The model under review builds one solid part; all positions refer to its coordinate system, in mm. Face numbers are marked on the shaded views. A direction names the side the tool comes from. Coordinates: 2 decimals unless noted, no trailing zeros. Order: outer loops, then holes, each group sorted by start corner. A loop starts at its lowest first (then second) coordinate and runs counter-clockwise, first axis right, second up. Notation, with made-up numbers: M 0,9 L 31,9 A31 ccw 31,35 Z; hole C 8,24.5 d1. An arc over 180 degrees is marked long. Answer as CSV lines item,"result". Start each with the question number.
Q1. Wall thickness on L1, parallel to Z at x = 194, y = 0; L2, parallel to Y at x = 96.5, z = 0; L3, parallel to Y at x = 192, z = -89.5: over which ranges is each line inside the solid? List them lowest first. Write a range as [from, to].
Q2. Consider section A-A on x = 111. Write out the cut boundary in (y, z).
Q3. Consider section B-B on z = -43. Write out the cut boundary in (x, y).
Q4. Machinability: for the marked faces 1 and 2, which of the approach directions +Z, -Z, +X, -X, +Y, -Y give a long, thin tool a straight path to every point of the face, cutting with its end or side? Answer none if there is none.
Q5. For P1, Ø1.5, axis at x = 252, z = -20, coming from the -Y side; P2, Ø2, axis at x = 225, y = -4.5, coming from the +Z side; P3, Ø1.5, axis at x = 195.5, y = -5, coming from the +Z side, all flat-tipped, find the tip position at first contact; note any pin that passes through.
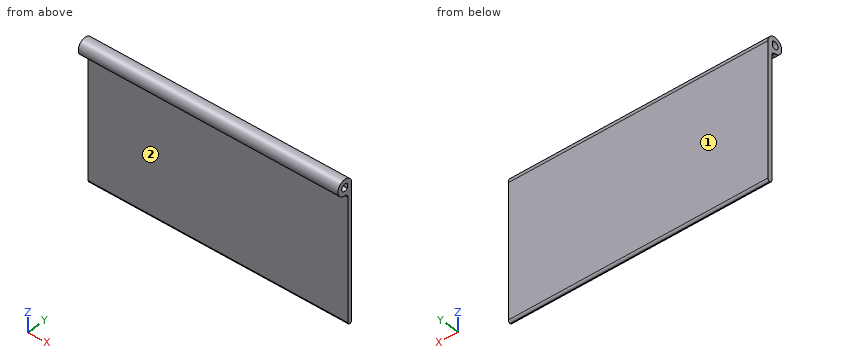
from build123d import *

# Parameters (mm, degrees)
SKETCH1_R               = 9
BOSS_EXTRUDE1_DEPTH     = 300
CUT_EXTRUDE1_DEPTH      = 301.269878609
CUT_EXTRUDE1_DEPTH_BACK = 301.269878609
BOSS_EXTRUDE2_START     = -300
BOSS_EXTRUDE2_DEPTH     = 300
CUT_EXTRUDE2_START      = -300
CUT_EXTRUDE2_DEPTH      = 300


# Read off the part's stored shape, not the designer's step: Cut-Extrude2
with BuildPart() as part:
    # Sketch1 → Boss-Extrude1 (new body)
    with BuildSketch(Plane(origin=(0, 0, 0), x_dir=(0, 0, -1), z_dir=(1, 0, 0))):
        Circle(SKETCH1_R)
    extrude(amount=BOSS_EXTRUDE1_DEPTH)

    # Sketch2 → Cut-Extrude1 (cut, two sides: drawn at the far end of the back side and taken through both)
    with BuildSketch(Plane(origin=(300, 0, 0), x_dir=(0, 0, -1), z_dir=(1, 0, 0)).offset(-CUT_EXTRUDE1_DEPTH_BACK)):
        with BuildLine():
            Line((-2.563201124, 3.2), (2.563201124, 3.2))
            ThreePointArc((2.563201124, 3.2), (0, -4.1), (-2.563201124, 3.2))
        make_face()
    extrude(amount=CUT_EXTRUDE1_DEPTH + CUT_EXTRUDE1_DEPTH_BACK, mode=Mode.SUBTRACT)

    # Sketch3 → Boss-Extrude2 (add)
    with BuildSketch(Plane(origin=(300, 0, 0), x_dir=(0, 0, -1), z_dir=(1, 0, 0)).offset(BOSS_EXTRUDE2_START)):
        with BuildLine():
            ThreePointArc((8.062257748, 4), (8.762428879, 2.054224947), (9, 0))
            ThreePointArc((9, 0), (10.171572875, 2.828427125), (13, 4))
            Line((13, 4), (8.062257748, 4))
        make_face()
        with BuildLine():
            ThreePointArc((5, 4), (7.828427125, 2.828427125), (9, 0))
            ThreePointArc((9, 0), (8.762428879, 2.054224947), (8.062257748, 4))
            Line((8.062257748, 4), (5, 4))
        make_face()
        with BuildLine():
            Line((154, 9), (0, 9))
            ThreePointArc((0, 9), (4.74341649, 7.64852927), (8.062257748, 4))
            Line((8.062257748, 4), (13, 4))
            Line((13, 4), (154, 4))
            Line((154, 4), (154, 9))
        make_face()
        with BuildLine():
            ThreePointArc((8.062257748, 4), (4.74341649, 7.64852927), (0, 9))
            Line((0, 9), (0, 4))
            Line((0, 4), (5, 4))
            Line((5, 4), (8.062257748, 4))
        make_face()
    extrude(amount=BOSS_EXTRUDE2_DEPTH)

    # Cut-Extrude2 outline → Cut-Extrude2 (cut)
    with BuildSketch(Plane(origin=(300, 0, 0), x_dir=(0, 0, -1), z_dir=(1, 0, 0)).offset(CUT_EXTRUDE2_START)):
        with BuildLine():
            ThreePointArc((151.5, 9), (153.267766953, 8.267766953), (154, 6.5))
            Line((154, 6.5), (154, 9))
            Line((154, 9), (151.5, 9))
        make_face()
        with BuildLine():
            ThreePointArc((154, 6.5), (153.267766953, 4.732233047), (151.5, 4))
            Line((151.5, 4), (154, 4))
            Line((154, 4), (154, 6.5))
        make_face()
    extrude(amount=CUT_EXTRUDE2_DEPTH, mode=Mode.SUBTRACT)


solid = part.part
Evaluation:
1,L1,"z = [-9, -4.1], [4.1, 9]"
1,L2,"y = [-9, -4.1], [3.2, 9]"
1,L3,"y = [4, 9]"
2,outline,"M 0,-9 A4 cw 4,-13 L 4,-151.5 A2.5 ccw 9,-151.5 L 9,0 A9 ccw long Z; hole M 3.2,-2.56 L 3.2,2.56 A4.1 ccw long Z"
3,outline,"M 0,4 L 300,4 L 300,9 L 0,9 Z"
4,face 1,"+Z, -Z, +X, -X, +Y"
4,face 2,"-Z, +X, -X, -Y"
5,P1,"stops at y = 4"
5,P2,"stops at z = 8.29"
5,P3,"stops at z = 7.93"
